Design review of the part built by this model. Coordinates are the model's own, in mm. Face numbers are marked on the shaded views. A direction names the side the tool comes from. Give positions to 0.01 mm unless a question says otherwise; leave off trailing zeros. Order: outer loops, then holes, each group sorted by start corner. A loop starts at its lowest first (then second) coordinate and runs counter-clockwise, first axis right, second up. Notation, with made-up numbers: M 51.25,28.25 L 85.25,28.25 A35 cw 85.25,62.25 Z; hole C 86.5,17 d1. An arc over 180 degrees is marked long. Answer as a JSON object with one key per item and string values.
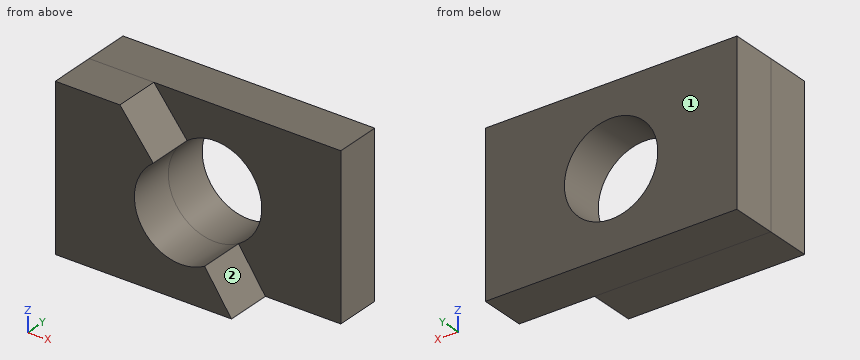
from build123d import *

# Parameters (mm, degrees)
F0_W     = 69.85
F0_H     = 44.45
F1_DEPTH = 12.7
F2_R     = 12.9689795612
F3_DEPTH = 25.4
F5_DEPTH = 12.7


with BuildPart() as f1:
    # F0 (on Front) → F1 (new body)
    with BuildSketch(Plane.XZ):
        with Locations((34.925, 22.225)):
            Rectangle(F0_W, F0_H)
    extrude(amount=F1_DEPTH)

    # F2 (on face) → F3 (cut)
    with BuildSketch(Plane.XZ.offset(12.7)):
        with Locations((34.925, 22.225)):
            Circle(F2_R)
    extrude(amount=-F3_DEPTH, mode=Mode.SUBTRACT)

    # F4 (on face) → F5 (join)
    with BuildSketch(Plane.XZ.offset(12.7)):
        with BuildLine():
            Line((27.1838563224, 32.6302450918), (17.9519541562, 44.45))
            Line((17.9519541562, 44.45), (0, 44.45))
            Line((0, 44.45), (0, 0))
            Line((0, 0), (48.9035993814, 0))
            Line((48.9035993814, 0), (41.4478117951, 11.0157468071))
            ThreePointArc((41.4478117951, 11.0157468071), (24.1005962211, 15.081701484), (27.1838563224, 32.6302450918))
        make_face()
    extrude(amount=F5_DEPTH)


solid = f1.part
(1) Insertion check: pin 1 (1.5 mm diameter, centred on y = -22, z = 9, fed in from +X); pin 2 (12 mm diameter, centred on x = 38, z = 13.5, fed in from -Y); pin 3 (5 mm diameter, centred on x = 59, z = 37.5, fed in from -Y). Each pin has a flat end and moves straight along its axis. Give the tip position at first contact, or say it passes through.
Checked values:
{"pin 1": "stops at x = 43.32", "pin 2": "stops at y = -25.4", "pin 3": "stops at y = -12.7"}
(2) We need section A-A (x = 34.5). Write out the cut boundary in (y, z), plus the area to 3 significant figures.
Checked values:
{"outline": "M -25.4,0 L 0,0 L 0,9.26 L -25.4,9.26 Z; M -12.7,35.19 L 0,35.19 L 0,44.45 L -12.7,44.45 Z", "area": "353 mm^2"}
(3) We need section B-B (z = 14). Write out the cut boundary in (x, y), plus the area to 3 significant figures.
Checked values:
{"outline": "M 0,-25.4 L 24.9,-25.4 L 24.9,0 L 0,0 Z; M 44.95,-12.7 L 69.85,-12.7 L 69.85,0 L 44.95,0 Z", "area": "949 mm^2"}
(4) Tool access review of the marked faces 1 and 2: name each direction out of +Z, -Z, +X, -X, +Y, -Y from which nothing blocks a thin tool from reaching the whole face with its end or side.
Checked values:
{"face 1": "+Z, -Z, +X, -X, +Y", "face 2": "+Z, +X, -Y"}
(5) To check wall thickness, follow L1, parallel to Y at x = 64.5, z = 29; L2, parallel to X at y = -6.75, z = 18.5; L3, parallel to X at y = -4.75, z = 15. State the ranges of each line that lie inside material, in increasing order. Write a range as from..to.
Checked values:
{"L1": "y = -12.7..0", "L2": "x = 0..22.5, 47.35..69.85", "L3": "x = 0..24.15, 45.7..69.85"}
(6) We need section D-D (z = 36.5). Write out the cut boundary in (x, y), plus the area to 3 significant figures.
Checked values:
{"outline": "M 0,-25.4 L 24.16,-25.4 L 24.16,-12.7 L 69.85,-12.7 L 69.85,0 L 0,0 Z", "area": "1,190 mm^2"}
(7) We need section C-C (y = -21). Write out the cut boundary in (x, z) (3 decimals), plus the area to 3 significant figures.
Checked values:
{"outline": "M 0,0 L 48.904,0 L 41.448,11.016 A12.969 cw 27.184,32.63 L 17.952,44.45 L 0,44.45 Z", "area": "1,260 mm^2"}
